Check sheet for the drawn part. Datum: minimum x, y, z corner. Units: mm. Give positions to 0.01 mm unless a question says otherwise; leave off trailing zeros. Write each loop counter-clockwise with the first axis right and the second up, starting at its lowest first coordinate (ties: lowest second). Pieces come first, ordered by that corner, then holes. Notation, with made-up numbers: M 38.25,25 L 90.25,25 A12 ccw 90.25,41 Z; hole C -35.5,-33 d7. An arc over 180 degrees is marked long. Write item = value, one per line. Start each with the question number.
1) Scan lines: L1, parallel to X at y = 1.4, z = 190; L2, parallel to Z at x = 80, y = 1.5; L3, parallel to Z at x = 169, y = 2.2. Record each from-to range of solid material in increasing order.
2) Gauge pin test, flat ends, axial feed: pin 1 (1.5 mm diameter, centred on y = 1.5, z = 133, fed in from +X); pin 2 (1.8 mm diameter, centred on x = 20, z = 50, fed in from -Y). Record the tip position at first contact, or that the pin passes through.
3) Sectioned sample at B-B, the plane x = 136.5. Record the cut outline in (y, z), then the cut area to 3 significant figures.
4) Sectioned sample at A-A, the plane y = 1.7. Count the separate pieces of the cut face and the enclosed holes in it, then the cut area to 3 significant figures.
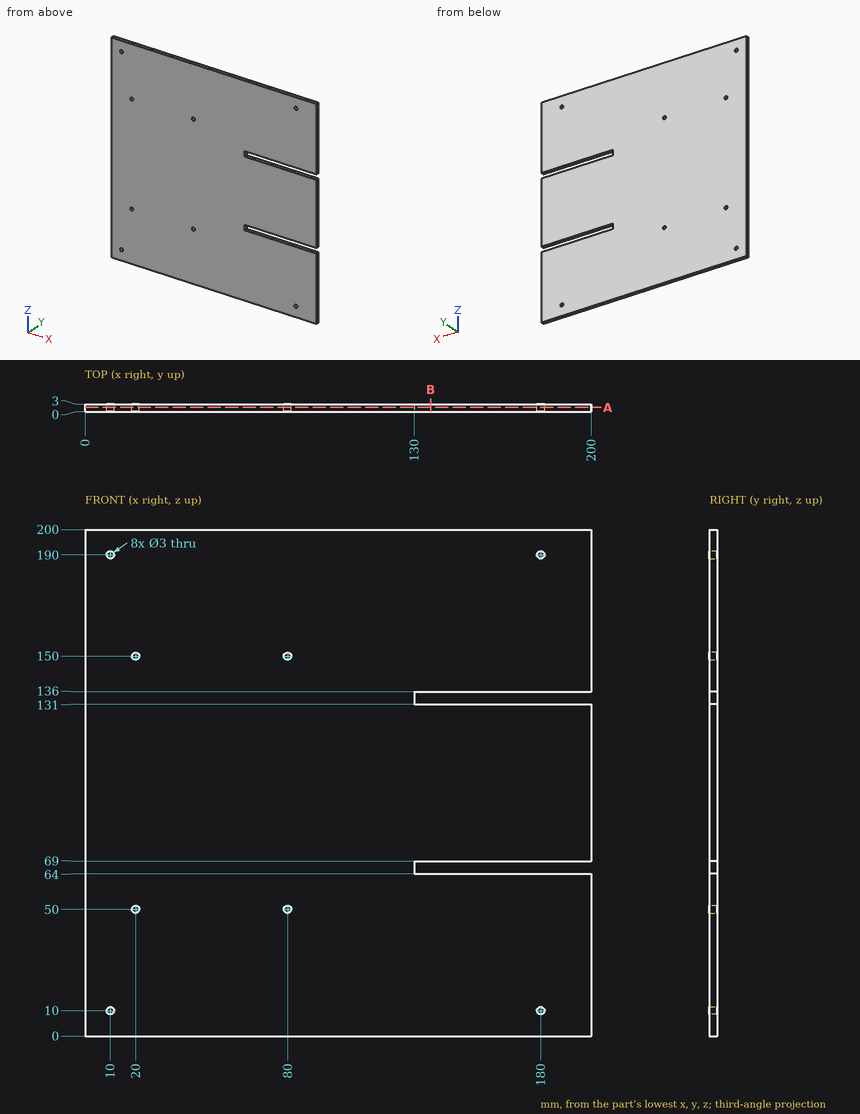
Data:
q1.L1 = 0 to 8.5, 11.5 to 178.5, 181.5 to 200
q1.L2 = 0 to 48.5, 51.5 to 148.5, 151.5 to 200
q1.L3 = 0 to 64, 69 to 131, 136 to 200
q2.pin_1 = 130
q2.pin_2 = through
q3.outline = M 0,0 L 3,0 L 3,64 L 0,64 Z; M 0,69 L 3,69 L 3,131 L 0,131 Z; M 0,136 L 3,136 L 3,200 L 0,200 Z
q3.area = 570 mm2
q4.separate_pieces = 1
q4.enclosed_holes = 8
q4.area = 39,200 mm2
